Here's the drawing with two shaded views (mm, measured from the low corner). I have some questions. A direction names the side the tool comes from. Give positions to 0.01 mm unless a question says otherwise; leave off trailing zeros. Loops run counter-clockwise (first coordinate to the right, second up) from the corner with the lowest first, then second, coordinate; pieces in that order, holes last.
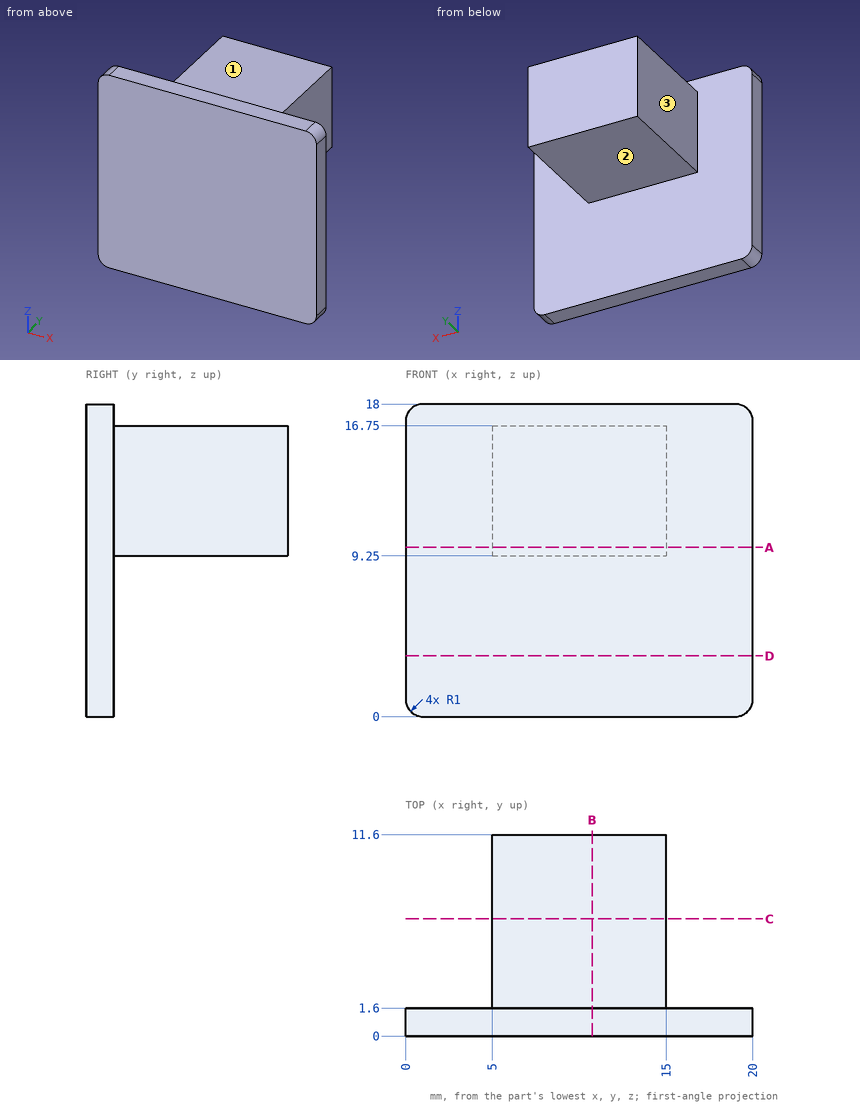
(1) Suppose I cut it at C-C on y = 6.75. List the corners of the cut face in (x, z) for me, plus the area to 3 significant figures.
Returned:
outline: (5, 9.25) - (15, 9.25) - (15, 16.75) - (5, 16.75) - close
area: 75.0 mm2
(2) Suppose I cut it at D-D on z = 3.5. List the corners of the cut face in (x, y) for me, plus the area to 3 significant figures.
Returned:
outline: (0, 0) - (20, 0) - (20, 1.6) - (0, 1.6) - close
area: 32.0 mm2
(3) Will these pins go through, and if not, where does the flat tip stop? P1, Ø6, axis at x = 8.5, z = 14, coming from the -Y side; P2, Ø1.5, axis at x = 6, y = 8, coming from the +Z side; P3, Ø6, axis at x = 14.5, y = 7, coming from the -Z side; P4, Ø2.5, axis at y = 7, z = 12.5, coming from the +X side.
Returned:
P1: stops at y = 0
P2: stops at z = 16.75
P3: stops at z = 9.25
P4: stops at x = 15
(4) Please list where these lines run through material, in increasing order: probe 1 along Z at (x, y) = (6, 2.5); probe 2 along Y at (x, z) = (5.25, 5); probe 3 along X at (y, z) = (9.5, 11).
Returned:
probe 1: z = 9.25 to 16.75
probe 2: y = 0 to 1.6
probe 3: x = 5 to 15
(5) Which directions (+Z, -Z, +X, -X, +Y, -Y) give clear straight access to the entire face, cutting with the end or side of a thin tool? Please do the marked faces 1, 2 and 3.
Returned:
face 1: +Z, +X, -X, +Y
face 2: -Z, +X, -X, +Y
face 3: +Z, -Z, -X, +Y
(6) Suppose I cut it at B-B on x = 10.75. List the corners of the cut face in (y, z) for me, plus the area to 3 significant figures.
Returned:
outline: (0, 0) - (1.6, 0) - (1.6, 9.25) - (11.6, 9.25) - (11.6, 16.75) - (1.6, 16.75) - (1.6, 18) - (0, 18) - close
area: 104 mm2
(7) Suppose I cut it at A-A on z = 9.75. List the corners of the cut face in (x, y) for me.
Returned:
outline: (0, 0) - (20, 0) - (20, 1.6) - (15, 1.6) - (15, 11.6) - (5, 11.6) - (5, 1.6) - (0, 1.6) - close
